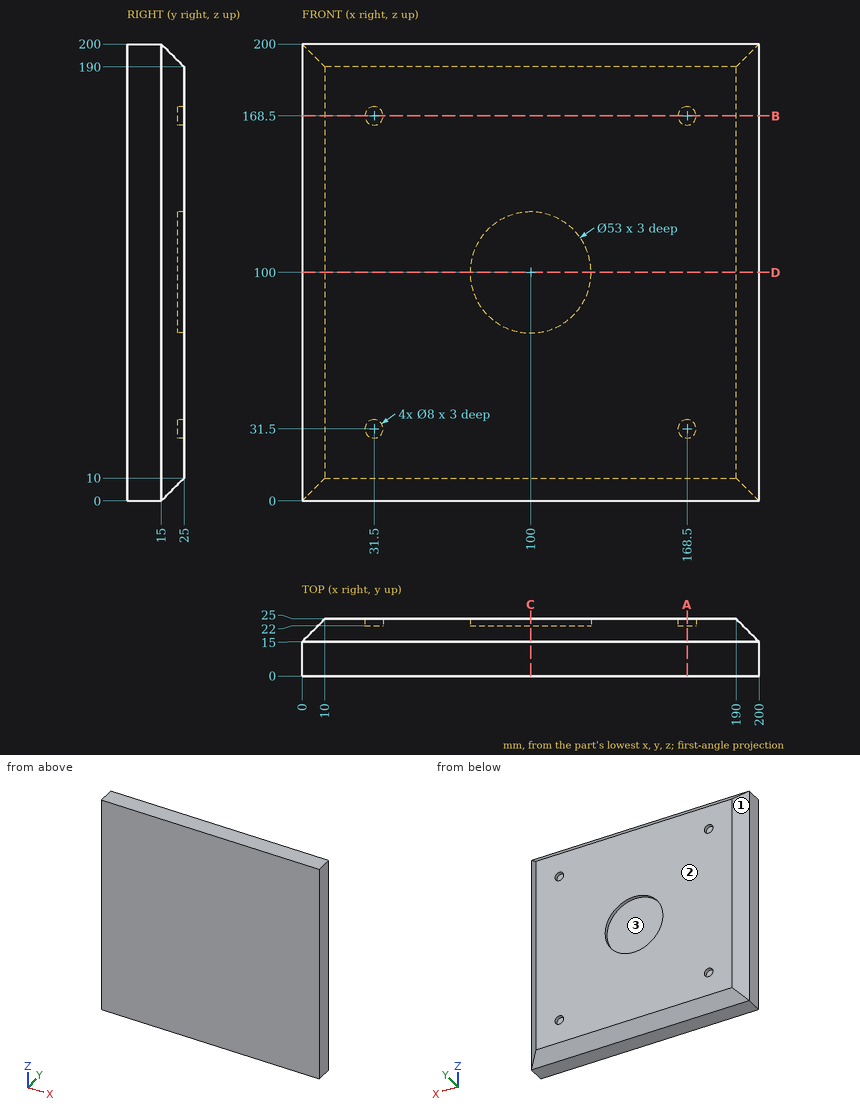
The figure shows three views and two pictorial views of one solid part (mm, origin at its lowest corner). Answer the questions. Round coordinates to 2 decimals unless told otherwise and drop trailing zeros. Write each loop counter-clockwise with the first axis right and the second up, starting at its lowest first coordinate (ties: lowest second). Pieces come first, ordered by that corner, then holes. Notation, with made-up numbers: (65.25, 61.5) -> (70.25, 61.5) arc R15 ccw to (70.25, 65.5) -> close; hole circle Ø6 at (-27.75, -18). An arc over 180 degrees is marked (long way). Write each question's results on one line, items separated by ' | '.
Q1. Section A-A, the plane x = 168.5 is taken. Write down the section's boundary in (y, z).
Data:
outline: (0, 0) -> (15, 0) -> (25, 10) -> (25, 27.5) -> (22, 27.5) -> (22, 35.5) -> (25, 35.5) -> (25, 164.5) -> (22, 164.5) -> (22, 172.5) -> (25, 172.5) -> (25, 190) -> (15, 200) -> (0, 200) -> close
Q2. Determine the mould class of the marked faces 1, 2 and 3 for opening direction X: released by +X, released by -X, zero draft, split by the parting line, or undercut.
Data:
face 1: released by -X | face 2: zero draft | face 3: undercut
Q3. Flat-ended cylindrical pins translate along their axes: P1, Ø6.5, axis at x = 169.5, z = 170.5, coming from the +Y side; P2, Ø5, axis at x = 168.5, z = 168.5, coming from the +Y side. Find the tip coordinate at first contact, or state that the pin passes through.
Data:
P1: y = 25 | P2: y = 22
Q4. Section C-C, the plane x = 100 is taken. Write down the section's boundary in (y, z), then the cut area to 3 significant figures.
Data:
outline: (0, 0) -> (15, 0) -> (25, 10) -> (25, 73.5) -> (22, 73.5) -> (22, 126.5) -> (25, 126.5) -> (25, 190) -> (15, 200) -> (0, 200) -> close | area: 4,740 mm^2
Q5. Straight lines are drawn through the part: line 1 along Y through (x, z) = (95.5, 116.5); line 2 along Z through (x, y) = (31.5, 22.7); line 3 along Z through (x, y) = (31.5, 23). For each, find the intervals that lie inside material, in ascending order. Write a range as [from, to].
Data:
line 1: [0, 22] | line 2: [7.7, 27.5], [35.5, 164.5], [172.5, 192.3] | line 3: [8, 27.5], [35.5, 164.5], [172.5, 192]
Q6. Section B-B, the plane z = 168.5 is taken. Write down the section's boundary in (x, y).
Data:
outline: (0, 0) -> (200, 0) -> (200, 15) -> (190, 25) -> (172.5, 25) -> (172.5, 22) -> (164.5, 22) -> (164.5, 25) -> (35.5, 25) -> (35.5, 22) -> (27.5, 22) -> (27.5, 25) -> (10, 25) -> (0, 15) -> close
Q7. Section D-D, the plane z = 100 is taken. Write down the section's boundary in (x, y).
Data:
outline: (0, 0) -> (200, 0) -> (200, 15) -> (190, 25) -> (126.5, 25) -> (126.5, 22) -> (73.5, 22) -> (73.5, 25) -> (10, 25) -> (0, 15) -> close
